The model under review builds one solid part; all positions refer to its coordinate system, in mm. Face numbers are marked on the shaded views. A direction names the side the tool comes from. Round coordinates to 2 decimals unless told otherwise and drop trailing zeros. Order: outer loops, then holes, each group sorted by start corner. A loop starts at its lowest first (then second) coordinate and runs counter-clockwise, first axis right, second up.
from build123d import *

# Parameters (mm, degrees)
BOX025_W                  = 1
BOX025_H                  = 1
BOX025_DEPTH              = 2
BOX027_W                  = 10
BOX027_H                  = 10
BOX027_DEPTH              = 10
BOX024_W                  = 10
BOX024_H                  = 10
BOX024_DEPTH              = 10
BOX017_W                  = 1
BOX017_H                  = 1
BOX017_DEPTH              = 2
BOX018_W                  = 1
BOX018_H                  = 1
BOX018_DEPTH              = 2
BOX019_W                  = 4
BOX019_H                  = 1
BOX019_DEPTH              = 2
BOX020_W                  = 1
BOX020_H                  = 1
BOX020_DEPTH              = 2
BOX021_W                  = 1
BOX021_H                  = 1
BOX021_DEPTH              = 2
BOX022_W                  = 4
BOX022_H                  = 1
BOX022_DEPTH              = 2
BOX023_W                  = 3.5
BOX023_H                  = 1
BOX023_DEPTH              = 2
BOX016_W                  = 1
BOX016_H                  = 1
BOX016_DEPTH              = 2
BOX015_W                  = 7
BOX015_H                  = 10
BOX015_DEPTH              = 2
BOX028_W                  = 1
BOX028_H                  = 1
BOX028_DEPTH              = 2
BOX026_W                  = 1
BOX026_H                  = 1
BOX026_DEPTH              = 2
BOX029_W                  = 2.5
BOX029_H                  = 1
BOX029_DEPTH              = 2
FUSION001_PLACEMENT_ANGLE = 180
BOX010_W                  = 1
BOX010_H                  = 1
BOX010_DEPTH              = 2
BOX012_W                  = 10
BOX012_H                  = 10
BOX012_DEPTH              = 10
BOX009_W                  = 10
BOX009_H                  = 10
BOX009_DEPTH              = 10
BOX002_W                  = 1
BOX002_H                  = 1
BOX002_DEPTH              = 2
BOX003_W                  = 1
BOX003_H                  = 1
BOX003_DEPTH              = 2
BOX004_W                  = 4
BOX004_H                  = 1
BOX004_DEPTH              = 2
BOX005_W                  = 1
BOX005_H                  = 1
BOX005_DEPTH              = 2
BOX006_W                  = 1
BOX006_H                  = 1
BOX006_DEPTH              = 2
BOX007_W                  = 4
BOX007_H                  = 1
BOX007_DEPTH              = 2
BOX008_W                  = 3.5
BOX008_H                  = 1
BOX008_DEPTH              = 2
BOX001_W                  = 1
BOX001_H                  = 1
BOX001_DEPTH              = 2
BOX_W                     = 7
BOX_H                     = 10
BOX_DEPTH                 = 2
BOX013_W                  = 1
BOX013_H                  = 1
BOX013_DEPTH              = 2
BOX011_W                  = 1
BOX011_H                  = 1
BOX011_DEPTH              = 2
BOX014_W                  = 2.5
BOX014_H                  = 1
BOX014_DEPTH              = 2
CYLINDER_R                = 10
CYLINDER_DEPTH            = 0.5


with BuildPart() as cubo025:
    # Box025 → Box025 (new body)
    with BuildSketch(Plane(origin=(-5, 3, 0), x_dir=(1, 0, 0), z_dir=(0, 0, 1))):
        with Locations((0.5, 0.5)):
            Rectangle(BOX025_W, BOX025_H)
    extrude(amount=BOX025_DEPTH)


with BuildPart() as cubo027:
    # Box027 → Box027 (new body)
    with BuildSketch(Plane(origin=(-15, 1, 0), x_dir=(1, 0, 0), z_dir=(0, 0, 1))):
        with Locations((5, 5)):
            Rectangle(BOX027_W, BOX027_H)
    extrude(amount=BOX027_DEPTH)


with BuildPart() as cubo024:
    # Box024 → Box024 (new body)
    with BuildSketch(Plane(origin=(-4, 3, 0), x_dir=(1, 0, 0), z_dir=(0, 0, 1))):
        with Locations((5, 5)):
            Rectangle(BOX024_W, BOX024_H)
    extrude(amount=BOX024_DEPTH)


with BuildPart() as cubo017:
    # Box017 → Box017 (new body)
    with BuildSketch(Plane(origin=(-3, 0, 0), x_dir=(1, 0, 0), z_dir=(0, 0, 1))):
        with Locations((0.5, 0.5)):
            Rectangle(BOX017_W, BOX017_H)
    extrude(amount=BOX017_DEPTH)


with BuildPart() as cubo018:
    # Box018 → Box018 (new body)
    with BuildSketch(Plane(origin=(-5, 2, 0), x_dir=(1, 0, 0), z_dir=(0, 0, 1))):
        with Locations((0.5, 0.5)):
            Rectangle(BOX018_W, BOX018_H)
    extrude(amount=BOX018_DEPTH)


with BuildPart() as cubo019:
    # Box019 → Box019 (new body)
    with BuildSketch(Plane(origin=(-5.5, -1, 0), x_dir=(0, -1, 0), z_dir=(0, 0, 1))):
        with Locations((2, 0.5)):
            Rectangle(BOX019_W, BOX019_H)
    extrude(amount=BOX019_DEPTH)


with BuildPart() as cubo020:
    # Box020 → Box020 (new body)
    with BuildSketch(Plane(origin=(-5, 4, 0), x_dir=(1, 0, 0), z_dir=(0, 0, 1))):
        with Locations((0.5, 0.5)):
            Rectangle(BOX020_W, BOX020_H)
    extrude(amount=BOX020_DEPTH)


with BuildPart() as cubo021:
    # Box021 → Box021 (new body)
    with BuildSketch(Plane(origin=(-6, 1, 0), x_dir=(1, 0, 0), z_dir=(0, 0, 1))):
        with Locations((0.5, 0.5)):
            Rectangle(BOX021_W, BOX021_H)
    extrude(amount=BOX021_DEPTH)


with BuildPart() as cubo022:
    # Box022 → Box022 (new body)
    with BuildSketch(Plane(origin=(-4, 3, 0), x_dir=(1, 0, 0), z_dir=(0, 0, 1))):
        with Locations((2, 0.5)):
            Rectangle(BOX022_W, BOX022_H)
    extrude(amount=BOX022_DEPTH)


with BuildPart() as cubo023:
    # Box023 → Box023 (new body)
    with BuildSketch(Plane(origin=(-3.5, -5, 0), x_dir=(1, 0, 0), z_dir=(0, 0, 1))):
        with Locations((1.75, 0.5)):
            Rectangle(BOX023_W, BOX023_H)
    extrude(amount=BOX023_DEPTH)


with BuildPart() as cubo016:
    # Box016 → Box016 (new body)
    with BuildSketch(Plane(origin=(-7, 0, 0), x_dir=(1, 0, 0), z_dir=(0, 0, 1))):
        with Locations((0.5, 0.5)):
            Rectangle(BOX016_W, BOX016_H)
    extrude(amount=BOX016_DEPTH)


with BuildPart() as cut021:
    # Box015 → Box015 (new body)
    with BuildSketch(Plane(origin=(-7, -5, 0), x_dir=(1, 0, 0), z_dir=(0, 0, 1))):
        with Locations((3.5, 5)):
            Rectangle(BOX015_W, BOX015_H)
    extrude(amount=BOX015_DEPTH)

    # Cut011: cut Cubo016
    add(cubo016.part, mode=Mode.SUBTRACT)

    # Cut012: cut Cubo023
    add(cubo023.part, mode=Mode.SUBTRACT)

    # Cut013: cut Cubo022
    add(cubo022.part, mode=Mode.SUBTRACT)

    # Cut014: cut Cubo021
    add(cubo021.part, mode=Mode.SUBTRACT)

    # Cut015: cut Cubo020
    add(cubo020.part, mode=Mode.SUBTRACT)

    # Cut016: cut Cubo019
    add(cubo019.part, mode=Mode.SUBTRACT)

    # Cut017: cut Cubo018
    add(cubo018.part, mode=Mode.SUBTRACT)

    # Cut018: cut Cubo017
    add(cubo017.part, mode=Mode.SUBTRACT)

    # Cut019: cut Cubo024
    add(cubo024.part, mode=Mode.SUBTRACT)

    # Cut020: cut Cubo027
    add(cubo027.part, mode=Mode.SUBTRACT)

    # Cut021: cut Cubo025
    add(cubo025.part, mode=Mode.SUBTRACT)


with BuildPart() as cubo028:
    # Box028 → Box028 (new body)
    with BuildSketch(Plane(origin=(-4, 3, 0), x_dir=(1, 0, 0), z_dir=(0, 0, 1))):
        with Locations((0.5, 0.5)):
            Rectangle(BOX028_W, BOX028_H)
    extrude(amount=BOX028_DEPTH)


with BuildPart() as cubo026:
    # Box026 → Box026 (new body)
    with BuildSketch(Plane(origin=(-5, 4, 0), x_dir=(1, 0, 0), z_dir=(0, 0, 1))):
        with Locations((0.5, 0.5)):
            Rectangle(BOX026_W, BOX026_H)
    extrude(amount=BOX026_DEPTH)


with BuildPart() as fusion001:
    # Box029 → Box029 (new body)
    with BuildSketch(Plane(origin=(-3.5, -6, 0), x_dir=(1, 0, 0), z_dir=(0, 0, 1))):
        with Locations((1.25, 0.5)):
            Rectangle(BOX029_W, BOX029_H)
    extrude(amount=BOX029_DEPTH)

    # Fusion001: union Cut021, Cubo028, Cubo026
    add(cut021.part)
    add(cubo028.part)
    add(cubo026.part)


with BuildPart() as fusion001_1:
    # Fusion001 placement: moved
    add(fusion001.part.moved(Location((0, 0, 2))).rotate(Axis((0, 0, 2), (0, 1, 0)), FUSION001_PLACEMENT_ANGLE))


with BuildPart() as cubo010:
    # Box010 → Box010 (new body)
    with BuildSketch(Plane(origin=(-5, 3, 0), x_dir=(1, 0, 0), z_dir=(0, 0, 1))):
        with Locations((0.5, 0.5)):
            Rectangle(BOX010_W, BOX010_H)
    extrude(amount=BOX010_DEPTH)


with BuildPart() as cubo012:
    # Box012 → Box012 (new body)
    with BuildSketch(Plane(origin=(-15, 1, 0), x_dir=(1, 0, 0), z_dir=(0, 0, 1))):
        with Locations((5, 5)):
            Rectangle(BOX012_W, BOX012_H)
    extrude(amount=BOX012_DEPTH)


with BuildPart() as cubo009:
    # Box009 → Box009 (new body)
    with BuildSketch(Plane(origin=(-4, 3, 0), x_dir=(1, 0, 0), z_dir=(0, 0, 1))):
        with Locations((5, 5)):
            Rectangle(BOX009_W, BOX009_H)
    extrude(amount=BOX009_DEPTH)


with BuildPart() as cubo002:
    # Box002 → Box002 (new body)
    with BuildSketch(Plane(origin=(-3, 0, 0), x_dir=(1, 0, 0), z_dir=(0, 0, 1))):
        with Locations((0.5, 0.5)):
            Rectangle(BOX002_W, BOX002_H)
    extrude(amount=BOX002_DEPTH)


with BuildPart() as cubo003:
    # Box003 → Box003 (new body)
    with BuildSketch(Plane(origin=(-5, 2, 0), x_dir=(1, 0, 0), z_dir=(0, 0, 1))):
        with Locations((0.5, 0.5)):
            Rectangle(BOX003_W, BOX003_H)
    extrude(amount=BOX003_DEPTH)


with BuildPart() as cubo004:
    # Box004 → Box004 (new body)
    with BuildSketch(Plane(origin=(-5.5, -1, 0), x_dir=(0, -1, 0), z_dir=(0, 0, 1))):
        with Locations((2, 0.5)):
            Rectangle(BOX004_W, BOX004_H)
    extrude(amount=BOX004_DEPTH)


with BuildPart() as cubo005:
    # Box005 → Box005 (new body)
    with BuildSketch(Plane(origin=(-5, 4, 0), x_dir=(1, 0, 0), z_dir=(0, 0, 1))):
        with Locations((0.5, 0.5)):
            Rectangle(BOX005_W, BOX005_H)
    extrude(amount=BOX005_DEPTH)


with BuildPart() as cubo006:
    # Box006 → Box006 (new body)
    with BuildSketch(Plane(origin=(-6, 1, 0), x_dir=(1, 0, 0), z_dir=(0, 0, 1))):
        with Locations((0.5, 0.5)):
            Rectangle(BOX006_W, BOX006_H)
    extrude(amount=BOX006_DEPTH)


with BuildPart() as cubo007:
    # Box007 → Box007 (new body)
    with BuildSketch(Plane(origin=(-4, 3, 0), x_dir=(1, 0, 0), z_dir=(0, 0, 1))):
        with Locations((2, 0.5)):
            Rectangle(BOX007_W, BOX007_H)
    extrude(amount=BOX007_DEPTH)


with BuildPart() as cubo008:
    # Box008 → Box008 (new body)
    with BuildSketch(Plane(origin=(-3.5, -5, 0), x_dir=(1, 0, 0), z_dir=(0, 0, 1))):
        with Locations((1.75, 0.5)):
            Rectangle(BOX008_W, BOX008_H)
    extrude(amount=BOX008_DEPTH)


with BuildPart() as cubo001:
    # Box001 → Box001 (new body)
    with BuildSketch(Plane(origin=(-7, 0, 0), x_dir=(1, 0, 0), z_dir=(0, 0, 1))):
        with Locations((0.5, 0.5)):
            Rectangle(BOX001_W, BOX001_H)
    extrude(amount=BOX001_DEPTH)


with BuildPart() as cut010:
    # Box → Box (new body)
    with BuildSketch(Plane(origin=(-7, -5, 0), x_dir=(1, 0, 0), z_dir=(0, 0, 1))):
        with Locations((3.5, 5)):
            Rectangle(BOX_W, BOX_H)
    extrude(amount=BOX_DEPTH)

    # Cut: cut Cubo001
    add(cubo001.part, mode=Mode.SUBTRACT)

    # Cut001: cut Cubo008
    add(cubo008.part, mode=Mode.SUBTRACT)

    # Cut002: cut Cubo007
    add(cubo007.part, mode=Mode.SUBTRACT)

    # Cut003: cut Cubo006
    add(cubo006.part, mode=Mode.SUBTRACT)

    # Cut004: cut Cubo005
    add(cubo005.part, mode=Mode.SUBTRACT)

    # Cut005: cut Cubo004
    add(cubo004.part, mode=Mode.SUBTRACT)

    # Cut006: cut Cubo003
    add(cubo003.part, mode=Mode.SUBTRACT)

    # Cut007: cut Cubo002
    add(cubo002.part, mode=Mode.SUBTRACT)

    # Cut008: cut Cubo009
    add(cubo009.part, mode=Mode.SUBTRACT)

    # Cut009: cut Cubo012
    add(cubo012.part, mode=Mode.SUBTRACT)

    # Cut010: cut Cubo010
    add(cubo010.part, mode=Mode.SUBTRACT)


with BuildPart() as cubo013:
    # Box013 → Box013 (new body)
    with BuildSketch(Plane(origin=(-4, 3, 0), x_dir=(1, 0, 0), z_dir=(0, 0, 1))):
        with Locations((0.5, 0.5)):
            Rectangle(BOX013_W, BOX013_H)
    extrude(amount=BOX013_DEPTH)


with BuildPart() as cubo011:
    # Box011 → Box011 (new body)
    with BuildSketch(Plane(origin=(-5, 4, 0), x_dir=(1, 0, 0), z_dir=(0, 0, 1))):
        with Locations((0.5, 0.5)):
            Rectangle(BOX011_W, BOX011_H)
    extrude(amount=BOX011_DEPTH)


with BuildPart() as fusion002:
    # Box014 → Box014 (new body)
    with BuildSketch(Plane(origin=(-3.5, -6, 0), x_dir=(1, 0, 0), z_dir=(0, 0, 1))):
        with Locations((1.25, 0.5)):
            Rectangle(BOX014_W, BOX014_H)
    extrude(amount=BOX014_DEPTH)

    # Fusion: union Cut010, Cubo013, Cubo011
    add(cut010.part)
    add(cubo013.part)
    add(cubo011.part)

    # Fusion002: union Fusion001
    add(fusion001_1.part)


with BuildPart() as fusion002_1:
    # Fusion002 placement: moved
    add(fusion002.part.moved(Location((0, 1, 0))))


with BuildPart() as fusion003:
    # Cylinder → Cylinder (new body)
    with BuildSketch(Plane.XY):
        Circle(CYLINDER_R)
    extrude(amount=CYLINDER_DEPTH)

    # Fusion003: union Fusion002
    add(fusion002_1.part)


solid = fusion003.part
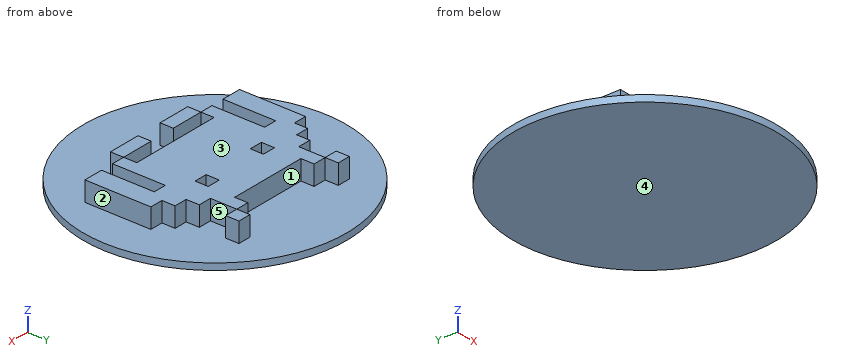
(1) We need section D-D (x = 3.75). Give the boundary of the cut face in (y, z), and give its area (3 significant figures).
(2) Tool access review of the marked faces 4 and 5: name each direction out of +Z, -Z, +X, -X, +Y, -Y from which nothing blocks a thin tool from reaching the whole face with its end or side.
(3) Clearance check with flat-ended pins moving along their axes: P1, Ø1.2, axis at x = -1.5, z = 1, coming from the -Y side; P2, Ø0.8, axis at x = -6.5, z = 1.5, coming from the +Y side; P3, Ø1.2, axis at y = 4, z = 1, coming from the -X side; P4, Ø6, axis at x = 4.5, y = -5, coming from the +Z side. State where each tip first meets the part, or that it passes through.
(4) We need section C-C (y = 8). Give the boundary of the cut face in (x, z), and give its area (3 significant figures).
(5) The part is to be moulded in two halves that separate along X. For the marked faces 1, 2 and 3, say which applies: pulls with the +X half, pulls with the -X half, needs draft (parallel to the pull), parting line crosses it, or undercut.
(6) We need section B-B (x = 0). Give the boundary of the cut face in (y, z), and give its area (3 significant figures).
(7) To check wall thickness, follow L1, parallel to X at y = 1.25, z = 1.9; L2, parallel to X at y = -0.25, z = 1; L3, parallel to Y at x = 1.25, z = 0.85. State the ranges of each line that lie inside material, in increasing order.
Verdict:
1. outline: (-9.27, 0) - (9.27, 0) - (9.27, 0.5) - (5, 0.5) - (5, 2) - (-4, 2) - (-4, 0.5) - (-9.27, 0.5) - close
1. area: 22.8 mm2
2. face 4: -Z, +X, -X, +Y, -Y
2. face 5: +Z, +X
3. P1: stops at y = -9.93
3. P2: stops at y = 1
3. P3: stops at x = -9.3
3. P4: stops at z = 2
4. outline: (-6, 0) - (6, 0) - (6, 0.5) - (-6, 0.5) - close
4. area: 6.00 mm2
5. face 1: undercut
5. face 2: pulls with the +X half
5. face 3: needs draft
6. outline: (-10, 0) - (10, 0) - (10, 0.5) - (4, 0.5) - (4, 2) - (-3, 2) - (-3, 0.5) - (-10, 0.5) - close
6. area: 20.5 mm2
7. L1: x = -6 to -3, -2 to 2, 3 to 6
7. L2: x = -7 to -5.5, -4.5 to 4.5, 5.5 to 7
7. L3: y = -5 to -4, -3 to 4
